from build123d import *

# Parameters (mm, degrees)
F0_R      = 44.45
F1_DEPTH  = 12.7
F2_R      = 19.05
F3_DEPTH  = 38.1
F4_R      = 9.525
F5_DEPTH  = 38.101
F7_DEPTH  = 38.101
F8_R      = 4.7625
F9_DEPTH  = 38.101
F10_R     = 44.45
F10_R_2   = 41.275
F11_DEPTH = 25.4


with BuildPart() as f1:
    # F0 (on Front) → F1 (new body)
    with BuildSketch(Plane.XZ):
        Circle(F0_R)
    extrude(amount=F1_DEPTH)

    # F2 (on Front) → F3 (join)
    with BuildSketch(Plane.XZ):
        Circle(F2_R)
    extrude(amount=F3_DEPTH)

    # F4 (on Front) → F5 (cut, through all)
    with BuildSketch(Plane.XZ):
        Circle(F4_R)
    extrude(amount=F5_DEPTH, mode=Mode.SUBTRACT)

    # F6 (on Front) → F7 (cut, through all)
    with BuildSketch(Plane.XZ):
        Polygon((-3.175, 0), (0, 0), (3.175, 0), (3.175, 12.7), (0, 12.7), (-3.175, 12.7), align=None)
    extrude(amount=F7_DEPTH, mode=Mode.SUBTRACT)

    # F8 (on Front) → F9 (cut, through all)
    with BuildSketch(Plane.XZ):
        with Locations((0, 28.575)):
            Circle(F8_R)
        with Locations((-24.746676, -14.2875)):
            Circle(F8_R)
        with Locations((24.746676, -14.2875)):
            Circle(F8_R)
    extrude(amount=F9_DEPTH, mode=Mode.SUBTRACT)

    # F10 (on Front) → F11 (join)
    with BuildSketch(Plane.XZ):
        Circle(F10_R)
        Circle(F10_R_2, mode=Mode.SUBTRACT)
    extrude(amount=F11_DEPTH)


solid = f1.part
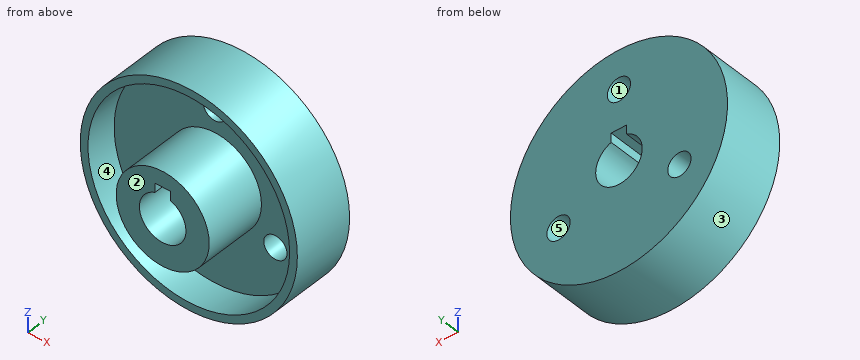
Check sheet for the modelled part. Datum: model origin and axes. Units: mm. Face numbers are marked on the shaded views. A direction names the side the tool comes from. Round coordinates to 2 decimals unless told otherwise and drop trailing zeros. Loops run counter-clockwise (first coordinate to the right, second up) from the corner with the lowest first, then second, coordinate; pieces in that order, holes last. Notation, with made-up numbers: (49, 41) -> (92, 41) arc R36 cw to (92, 78) -> close; hole circle Ø8 at (-35.75, 1.25). An arc over 180 degrees is marked (long way). Put each result on its own line as item: value. Start each with the question number.
1. Access from +Z, -Z, +X, -X, +Y, -Y to the whole of each face (thin tool, end or side, straight path). Record for the marked faces 4 and 5.
2. Gauge pin test, flat ends, axial feed: pin 1 (6 mm diameter, centred on x = -27, y = -7.5, fed in from -Z); pin 2 (3 mm diameter, centred on x = -1.5, y = -17, fed in from -Z); pin 3 (4 mm diameter, centred on x = -6.5, y = -16, fed in from -Z); pin 4 (8.5 mm diameter, centred on x = 24.75, z = -14.29, fed in from +Y). Record the tip position at first contact, or that the pin passes through.
3. Draft check along Z on the marked faces 1, 2 and 3. Enter one of: +Z half, -Z half, draft (parallel to the pull), parting line (faces both ways), or undercut.
4. Section check A-A (y = -19). Enter the section's corners in (x, z) (3 decimals), plus the area to 3 significant figures.
5. Section check B-B (x = 0). Give the number of separate pieces and of enclosed holes in the cut face, plus the area to 3 significant figures.
6. Scan lines: probe 1 along Z at (x, y) = (0, -21) (3 decimals); probe 2 along X at (y, z) = (-23, 13); probe 3 along Z at (x, y) = (-3, -3). Record each from-to range of solid material in increasing order.
7. Section check D-D (y = -28.5). Enter the section's corners in (x, z) (3 decimals).
8. Section check C-C (z = 0). Enter the section's corners in (x, y) (3 decimals).
Findings:
1. face 4: -Y
1. face 5: +Y, -Y
2. pin 1: stops at z = -37.41
2. pin 2: stops at z = -44.45
2. pin 3: stops at z = -44.22
2. pin 4: passes through
3. face 1: undercut
3. face 2: draft
3. face 3: parting line
4. outline: circle Ø88.9 at (0, 0); circle Ø38.1 at (0, 0); hole circle Ø82.55 at (0, 0); hole (-3.175, 8.98) arc R9.525 ccw (long way) to (3.175, 8.98) -> (3.175, 12.7) -> (-3.175, 12.7) -> close
4. area: 1,690 mm^2
5. separate pieces: 3
5. enclosed holes: 0
5. area: 1,210 mm^2
6. probe 1: z = -44.45 to -41.275, -19.05 to -9.525, 12.7 to 19.05, 41.275 to 44.45
6. probe 2: x = -42.51 to -39.17, -13.92 to 13.92, 39.17 to 42.51
6. probe 3: z = -44.35 to -9.04, 12.7 to 24.88, 32.27 to 44.35
7. outline: circle Ø38.1 at (0, 0); hole (-3.175, 8.98) arc R9.525 ccw (long way) to (3.175, 8.98) -> (3.175, 12.7) -> (-3.175, 12.7) -> close
8. outline: (-44.45, -25.4) -> (-41.275, -25.4) -> (-41.275, -12.7) -> (-19.05, -12.7) -> (-19.05, -38.1) -> (-9.525, -38.1) -> (-9.525, 0) -> (-44.45, 0) -> close; (9.525, -38.1) -> (19.05, -38.1) -> (19.05, -12.7) -> (41.275, -12.7) -> (41.275, -25.4) -> (44.45, -25.4) -> (44.45, 0) -> (9.525, 0) -> close
